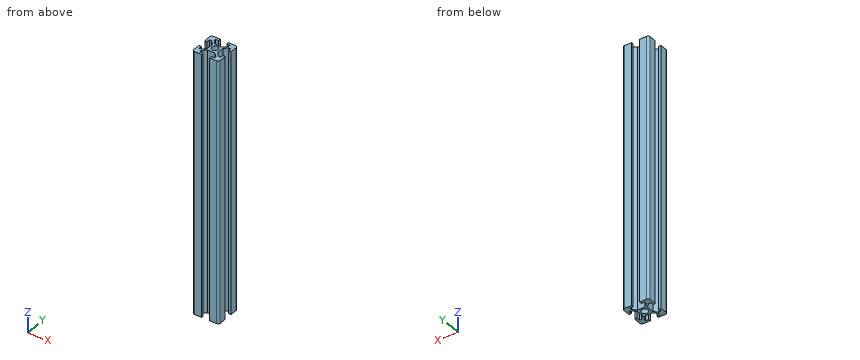
from build123d import *

# Parameters (mm, degrees)
SKETCH1_R           = 2.5
BOSS_EXTRUDE1_DEPTH = 200


with BuildPart() as part:
    # Sketch1 → Boss-Extrude1 (new body)
    with BuildSketch(Plane.XY):
        with BuildLine():
            Line((2.839339828, 3.9), (5.5, 6.560660172))
            Line((5.5, 6.560660172), (5.5, 8.2))
            Line((5.5, 8.2), (3.1, 8.2))
            Line((3.1, 8.2), (3.1, 10))
            Line((3.1, 10), (8.5, 10))
            ThreePointArc((8.5, 10), (9.560660172, 9.560660172), (10, 8.5))
            Line((10, 8.5), (10, 3.1))
            Line((10, 3.1), (8.2, 3.1))
            Line((8.2, 3.1), (8.2, 5.5))
            Line((8.2, 5.5), (6.560660172, 5.5))
            Line((6.560660172, 5.5), (3.9, 2.839339828))
            Line((3.9, 2.839339828), (3.9, -2.839339828))
            Line((3.9, -2.839339828), (6.560660172, -5.5))
            Line((6.560660172, -5.5), (8.2, -5.5))
            Line((8.2, -5.5), (8.2, -3.1))
            Line((8.2, -3.1), (10, -3.1))
            Line((10, -3.1), (10, -8.5))
            ThreePointArc((10, -8.5), (9.560660172, -9.560660172), (8.5, -10))
            Line((8.5, -10), (3.1, -10))
            Line((3.1, -10), (3.1, -8.2))
            Line((3.1, -8.2), (5.5, -8.2))
            Line((5.5, -8.2), (5.5, -6.560660172))
            Line((5.5, -6.560660172), (2.839339828, -3.9))
            Line((2.839339828, -3.9), (-2.839339828, -3.9))
            Line((-2.839339828, -3.9), (-5.5, -6.560660172))
            Line((-5.5, -6.560660172), (-5.5, -8.2))
            Line((-5.5, -8.2), (-3.1, -8.2))
            Line((-3.1, -8.2), (-3.1, -10))
            Line((-3.1, -10), (-8.5, -10))
            ThreePointArc((-8.5, -10), (-9.560660172, -9.560660172), (-10, -8.5))
            Line((-10, -8.5), (-10, -3.1))
            Line((-10, -3.1), (-8.2, -3.1))
            Line((-8.2, -3.1), (-8.2, -5.5))
            Line((-8.2, -5.5), (-6.560660172, -5.5))
            Line((-6.560660172, -5.5), (-3.9, -2.839339828))
            Line((-3.9, -2.839339828), (-3.9, 2.839339828))
            Line((-3.9, 2.839339828), (-6.560660172, 5.5))
            Line((-6.560660172, 5.5), (-8.2, 5.5))
            Line((-8.2, 5.5), (-8.2, 3.1))
            Line((-8.2, 3.1), (-10, 3.1))
            Line((-10, 3.1), (-10, 8.5))
            ThreePointArc((-10, 8.5), (-9.560660172, 9.560660172), (-8.5, 10))
            Line((-8.5, 10), (-3.1, 10))
            Line((-3.1, 10), (-3.1, 8.2))
            Line((-3.1, 8.2), (-5.5, 8.2))
            Line((-5.5, 8.2), (-5.5, 6.560660172))
            Line((-5.5, 6.560660172), (-2.839339828, 3.9))
            Line((-2.839339828, 3.9), (2.839339828, 3.9))
        make_face()
        with Locations((0, 0.235847297)):
            Circle(SKETCH1_R, mode=Mode.SUBTRACT)
    extrude(amount=BOSS_EXTRUDE1_DEPTH)


solid = part.part
Verification items for the finished model (mm, model axes). Give positions to 0.01 mm unless a question says otherwise; leave off trailing zeros. Loops run counter-clockwise (first coordinate to the right, second up) from the corner with the lowest first, then second, coordinate; pieces in that order, holes last.
1. Go/stop test with flat-tipped pins: P1, Ø1.7, axis at x = 1, z = 118, coming from the +Y side; P2, Ø3, axis at y = 1, z = 73, coming from the +X side; P3, Ø0.5, axis at y = 9.5, z = 119, coming from the +X side. Record where each tip stops, or that it passes through.
Derived:
P1: stops at y = 3.9
P2: stops at x = 3.9
P3: stops at x = 9.8
2. Material ranges on probe 1 along X at (y, z) = (-3.25, 83.5); probe 2 along Y at (x, z) = (-4.5, 84); probe 3 along X at (y, z) = (8, 123.5), recorded low to high.
Derived:
probe 1: x = -10 to -8.2, -4.31 to 4.31, 8.2 to 10
probe 2: y = -10 to -8.2, -5.56 to -3.44, 3.44 to 5.56, 8.2 to 10
probe 3: x = -10 to -5.5, 5.5 to 10
3. Cross-section at A-A on x = 0. Record the cut outline in (y, z), and give its area (3 significant figures).
Derived:
outline: (-3.9, 0) - (-2.26, 0) - (-2.26, 200) - (-3.9, 200) - close; (2.74, 0) - (3.9, 0) - (3.9, 200) - (2.74, 200) - close
area: 560 mm2
